For this review, take the finished solid that the model builds, in its own axes (mm). A direction names the side the tool comes from. Give positions to 0.01 mm unless a question says otherwise; leave off trailing zeros. Write each loop counter-clockwise with the first axis right and the second up, starting at its lowest first coordinate (ties: lowest second). Pieces come first, ordered by that corner, then holes. Notation, with made-up numbers: M 40,23 L 72,23 A20 cw 72,51 Z; hole C 3.5,-20.75 d7. An arc over 180 degrees is marked long. Write item = value, one per line.
```python
from build123d import *

# Parameters (mm, degrees)
BOSS_EXTRUDE1_DEPTH = 152.4


with BuildPart() as part:
    # Sketch2 → Boss-Extrude1 (new, symmetric)
    with BuildSketch(Plane.XY):
        with BuildLine():
            Line((-15.875, 0), (15.875, 0))
            Line((15.875, 0), (15.875, 31.75))
            Line((15.875, 31.75), (14.2875, 31.75))
            Line((14.2875, 31.75), (14.2875, 1.9685))
            ThreePointArc((14.2875, 1.9685), (14.175907684, 1.699092316), (13.9065, 1.5875))
            Line((13.9065, 1.5875), (-15.875, 1.5875))
            Line((-15.875, 1.5875), (-15.875, 0))
        make_face()
    extrude(amount=BOSS_EXTRUDE1_DEPTH, both=True)


solid = part.part
```
1. Machinability: for faces 1 (the face through (14.288, 17, 2)), 2 (the face through (0, 0, 2)), which of the approach directions +Z, -Z, +X, -X, +Y, -Y give a long, thin tool a straight path to every point of the face, cutting with its end or side? Answer none if there is none.
Responses:
face_1 = +Z, -Z, -X, +Y
face_2 = +Z, -Z, +X, -X, -Y
2. Insertion check: P1, Ø3, axis at y = 4, z = -1, coming from the -X side; P2, Ø15, axis at x = -1, z = -3, coming from the +Y side; P3, Ø8, axis at x = -0.5, y = 5, coming from the +Z side. Each pin has a flat end and moves straight along its axis. Give the tip position at first contact, or say it passes through.
Responses:
P1 = 14.29
P2 = 1.59
P3 = 152.4
3. We need section C-C, the plane y = 20. Write out the cut boundary in (x, z) (1 decimal), then the cut area to 3 significant figures.
Responses:
outline = M 14.3,-152.4 L 15.9,-152.4 L 15.9,152.4 L 14.3,152.4 Z
area = 484 mm2
4. We need section B-B, the plane x = -6.5. Write out the cut boundary in (y, z), then the cut area to 3 significant figures.
Responses:
outline = M 0,-152.4 L 1.59,-152.4 L 1.59,152.4 L 0,152.4 Z
area = 484 mm2
5. For line 1 along Y through (x, z) = (7, 44.5); line 2 along X through (y, z) = (24, 101.5) (1 decimal), list the stretches that pass through material, from the lowest coordinate up. Write a range as from..to.
Responses:
line_1 = 0..1.59
line_2 = 14.3..15.9
